```python
from build123d import *

# Parameters (mm, degrees)
ESQUISSE1_R             = 1.6
BOSS_EXTRU_1_DEPTH      = 10
ESQUISSE2_R             = 32.8
BOSS_EXTRU_2_DEPTH      = 22
ENL_V_MAT_EXTRU_1_DEPTH = 3.5
BOSS_EXTRU_3_REACH      = 79.261
ESQUISSE4_R             = 32.8
ESQUISSE5_R             = 16
BOSS_EXTRU_4_DEPTH      = 19
ESQUISSE6_R             = 1
BOSS_EXTRU_5_DEPTH      = 27
BOSS_EXTRU_6_DEPTH      = 1.5
ESQUISSE8_R             = 5
BOSS_EXTRU_7_DEPTH      = 5.5
SKETCH_1_W              = 183.813547174
SKETCH_1_H              = 124.067416174
CUT_EXTRUDE_1_DEPTH     = 18


with BuildPart() as part:
    # Esquisse1 → Boss.-Extru.1 (new body)
    with BuildSketch(Plane.XY):
        with BuildLine():
            ThreePointArc((-56.3, -16.861494596), (-60.528670487, -14.599558136), (-64.01, -11.301322931))
            ThreePointArc((-64.01, -11.301322931), (-65, 0), (-64.01, 11.301322931))
            ThreePointArc((-64.01, 11.301322931), (-60.528670487, 14.599558136), (-56.3, 16.861494596))
            Line((-56.3, 16.861494596), (-39.624688626, 23.091930519))
            ThreePointArc((-39.624688626, 23.091930519), (-36.690940127, 29.525679018), (-30.257191628, 26.591930519))
            Line((-30.257191628, 26.591930519), (-12.425, 33.254614341))
            ThreePointArc((-12.425, 33.254614341), (1.381675102, 35.473102119), (14.973963383, 32.187426436))
            Line((14.973963383, 32.187426436), (20.756023105, 34.801647207))
            ThreePointArc((20.756023105, 34.801647207), (24.347774736, 34.238511045), (26, 31))
            Line((26, 31), (25.359978077, 24.841930519))
            ThreePointArc((25.359978077, 24.841930519), (35.5, 0), (25.359978077, -24.841930519))
            Line((25.359978077, -24.841930519), (26, -31))
            ThreePointArc((26, -31), (24.347774736, -34.238511045), (20.756023105, -34.801647207))
            Line((20.756023105, -34.801647207), (14.973963383, -32.187426436))
            ThreePointArc((14.973963383, -32.187426436), (1.381675102, -35.473102119), (-12.425, -33.254614341))
            Line((-12.425, -33.254614341), (-30.257191628, -26.591930519))
            ThreePointArc((-30.257191628, -26.591930519), (-36.690940127, -29.525679018), (-39.624688626, -23.091930519))
            Line((-39.624688626, -23.091930519), (-56.3, -16.861494596))
        make_face()
        with Locations((-35, -25)):
            Circle(ESQUISSE1_R, mode=Mode.SUBTRACT)
        with Locations((22, 31)):
            Circle(ESQUISSE1_R, mode=Mode.SUBTRACT)
        with Locations((-35, 25)):
            Circle(ESQUISSE1_R, mode=Mode.SUBTRACT)
        with Locations((22, -31)):
            Circle(ESQUISSE1_R, mode=Mode.SUBTRACT)
    extrude(amount=BOSS_EXTRU_1_DEPTH)

    # Esquisse2 → Boss.-Extru.2 (add)
    with BuildSketch(Plane.XY.offset(10)):
        Circle(ESQUISSE2_R)
    extrude(amount=BOSS_EXTRU_2_DEPTH)

    # Esquisse3 → Enl_v. mat.-Extru.1 (cut)
    with BuildSketch(Plane.XY.offset(10)):
        with BuildLine():
            Line((-55.775, -15.456370046), (-37.378202776, -22.330008789))
            ThreePointArc((-37.378202776, -22.330008789), (-36.165940127, -28.120554469), (-31.453677478, -24.543603151))
            Line((-31.453677478, -24.543603151), (-11.9, -31.849489792))
            ThreePointArc((-11.9, -31.849489792), (1.664031028, -33.959255009), (14.956816294, -30.533484019))
            Line((14.956816294, -30.533484019), (21.291141631, -33.397398551))
            ThreePointArc((21.291141631, -33.397398551), (23.468656713, -33.023128137), (24.499056843, -31.06866508))
            Line((24.499056843, -31.06866508), (23.79417774, -24.286562245))
            ThreePointArc((23.79417774, -24.286562245), (34, 0), (23.79417774, 24.286562245))
            Line((23.79417774, 24.286562245), (24.499056843, 31.06866508))
            ThreePointArc((24.499056843, 31.06866508), (23.468656713, 33.023128137), (21.291141631, 33.397398551))
            Line((21.291141631, 33.397398551), (14.956816294, 30.533484019))
            ThreePointArc((14.956816294, 30.533484019), (1.664031028, 33.959255009), (-11.9, 31.849489792))
            Line((-11.9, 31.849489792), (-31.453677478, 24.543603151))
            ThreePointArc((-31.453677478, 24.543603151), (-36.165940127, 28.120554469), (-37.378202776, 22.330008789))
            Line((-37.378202776, 22.330008789), (-55.775, 15.456370046))
            ThreePointArc((-55.775, 15.456370046), (-59.496201473, 13.493411636), (-62.6, 10.653168543))
            ThreePointArc((-62.6, 10.653168543), (-63.5, 0), (-62.6, -10.653168543))
            ThreePointArc((-62.6, -10.653168543), (-59.496201473, -13.493411636), (-55.775, -15.456370046))
        make_face()
    extrude(amount=-ENL_V_MAT_EXTRU_1_DEPTH, mode=Mode.SUBTRACT)


with BuildPart() as enl_v_mat_extru_1_piece_1:
    # of the separate pieces the step leaves, piece 1, a body of its own (enl_v_mat_extru_1_pieces)
    add(part.part.solids().sort_by_distance((32.8, 0, 10))[0])


with BuildPart() as enl_v_mat_extru_1_piece_2:
    # of the separate pieces the step leaves, piece 2, a body of its own (enl_v_mat_extru_1_pieces)
    add(part.part.solids().sort_by_distance((-64.01, 11.301322931, 0))[0])

    # Esquisse4 → Boss.-Extru.3 (add, up to next)
    with BuildSketch(Plane(origin=(0, 0, 10), x_dir=(-1, 0, 0), z_dir=(0, 0, -1)), mode=Mode.PRIVATE) as boss_extru_3_sk1:
        with Locations(Location((0, 0, 0), (0, 0, 180))):
            Circle(ESQUISSE4_R)
    boss_extru_3_tool1 = extrude(boss_extru_3_sk1.sketch, amount=BOSS_EXTRU_3_REACH, mode=Mode.PRIVATE) - enl_v_mat_extru_1_piece_2.part

    add(enl_v_mat_extru_1_piece_1.part)  # Boss.-Extru.3 merges Enl_v. mat.-Extru.1 piece 1
    add(boss_extru_3_tool1.solids().sort_by_distance((0, 0, 10))[0])

    # Esquisse5 → Boss.-Extru.4 (add)
    with BuildSketch(Plane(origin=(0, 0, 0), x_dir=(-1, 0, 0), z_dir=(0, 0, -1))):
        with Locations(Location((50, 0, 0), (0, 0, 336.653490915))):
            Circle(ESQUISSE5_R)
    extrude(amount=BOSS_EXTRU_4_DEPTH)

    # Esquisse6 → Boss.-Extru.5 (add)
    # profile 1 of 4: a face of its own
    with BuildSketch(Plane(origin=(0, 0, 0), x_dir=(-1, 0, 0), z_dir=(0, 0, -1))):
        Polygon((-20.489225606, -29.008126327), (-22.969626005, -28.695694159), (-24.480400399, -30.687567832), (-23.510774394, -32.991873673), (-21.030373995, -33.304305841), (-19.519599601, -31.312432168), align=None)
        with Locations((-22, -31)):
            Circle(ESQUISSE6_R, mode=Mode.SUBTRACT)
    # profile 2 of 4: a face of its own
    with BuildSketch(Plane(origin=(0, 0, 0), x_dir=(-1, 0, 0), z_dir=(0, 0, -1))):
        Polygon((36.086835018, -22.748602735), (33.593650283, -22.933074633), (32.506815266, -25.184471898), (33.913164982, -27.251397265), (36.406349717, -27.066925367), (37.493184734, -24.815528102), align=None)
        with Locations((35, -25)):
            Circle(ESQUISSE6_R, mode=Mode.SUBTRACT)
    # profile 3 of 4: a face of its own
    with BuildSketch(Plane(origin=(0, 0, 0), x_dir=(-1, 0, 0), z_dir=(0, 0, -1))):
        Polygon((36.720274889, 26.814016072), (34.289153443, 27.396809791), (32.568878555, 25.582793719), (33.279725111, 23.185983928), (35.710846557, 22.603190209), (37.431121445, 24.417206281), align=None)
        with Locations((35, 25)):
            Circle(ESQUISSE6_R, mode=Mode.SUBTRACT)
    # profile 4 of 4: a face of its own
    with BuildSketch(Plane(origin=(0, 0, 0), x_dir=(-1, 0, 0), z_dir=(0, 0, -1))):
        Polygon((-19.952160425, 32.43399898), (-22.217959758, 33.490480585), (-24.265799333, 32.056481605), (-24.047839575, 29.56600102), (-21.782040242, 28.509519415), (-19.734200667, 29.943518395), align=None)
        with Locations((-22, 31)):
            Circle(ESQUISSE6_R, mode=Mode.SUBTRACT)
    extrude(amount=BOSS_EXTRU_5_DEPTH)

    # Esquisse7 → Boss.-Extru.6 (add)
    with BuildSketch(Plane(origin=(0, 0, -8), x_dir=(-1, 0, 0), z_dir=(0, 0, -1))):
        with BuildLine():
            Line((30.257191628, 26.591930519), (12.425, 33.254614341))
            ThreePointArc((12.425, 33.254614341), (-1.381675102, 35.473102119), (-14.973963383, 32.187426436))
            Line((-14.973963383, 32.187426436), (-20.756023105, 34.801647207))
            ThreePointArc((-20.756023105, 34.801647207), (-24.347774736, 34.238511045), (-26, 31))
            Line((-26, 31), (-25.359978077, 24.841930519))
            ThreePointArc((-25.359978077, 24.841930519), (-35.5, 0), (-25.359978077, -24.841930519))
            Line((-25.359978077, -24.841930519), (-26, -31))
            ThreePointArc((-26, -31), (-24.347774736, -34.238511045), (-20.756023105, -34.801647207))
            Line((-20.756023105, -34.801647207), (-14.973963383, -32.187426436))
            ThreePointArc((-14.973963383, -32.187426436), (-1.381675102, -35.473102119), (12.425, -33.254614341))
            Line((12.425, -33.254614341), (30.257191628, -26.591930519))
            ThreePointArc((30.257191628, -26.591930519), (36.690940127, -29.525679018), (39.624688626, -23.091930519))
            ThreePointArc((39.624688626, -23.091930519), (33.487603548, 0), (39.624688626, 23.091930519))
            ThreePointArc((39.624688626, 23.091930519), (36.690940127, 29.525679018), (30.257191628, 26.591930519))
        make_face()
    extrude(amount=BOSS_EXTRU_6_DEPTH)

    # Esquisse8 → Boss.-Extru.7 (add)
    with BuildSketch(Plane.XY.offset(6.5)):
        with Locations((-50, 0)):
            Circle(ESQUISSE8_R)
    extrude(amount=BOSS_EXTRU_7_DEPTH)

    # Sketch 1 → Cut-Extrude 1 (cut)
    with BuildSketch(Plane(origin=(0, 0, -19), x_dir=(-1, 0, 0), z_dir=(0, 0, -1))):
        with Locations((14.308056493, -2.422140446)):
            Rectangle(SKETCH_1_W, SKETCH_1_H)
    extrude(amount=CUT_EXTRUDE_1_DEPTH, mode=Mode.SUBTRACT)


solid = enl_v_mat_extru_1_piece_2.part
```
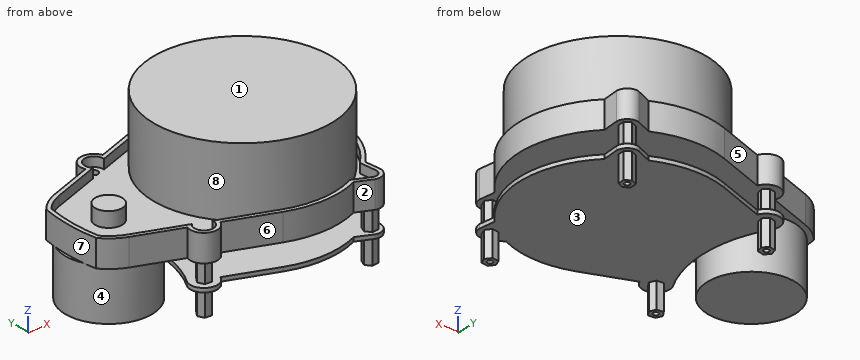
Can you work these out from the model? Positions are in its coordinate system, mm. Face numbers are marked on the shaded views. A direction names the side the tool comes from. Round coordinates to 2 decimals unless told otherwise and drop trailing zeros. Loops run counter-clockwise (first coordinate to the right, second up) from the corner with the lowest first, then second, coordinate; pieces in that order, holes last.
Item 1: Please list where these lines run through material, in increasing order: L1, parallel to Y at x = 22, z = 4; L2, parallel to Y at x = -35, z = 3.25; L3, parallel to Z at x = -27.5, y = 10.
Item 2: Suppose I cut it at A-A, the plane y = 0. Write out the boundary of the cut face in (x, z).
Item 3: Suppose I cut it at B-B, the plane x = 0.5. Write out the boundary of the cut face in (y, z), then the cut area to 3 significant figures.
Item 4: Which directions (+Z, -Z, +X, -X, +Y, -Y) give clear straight access to the entire face, cutting with the end or side of a thin tool? Please do the marked faces 4, 5, 6, 7 and 8.
Item 5: Will these pins go through, and if not, where does the flat tip stop? pin 1 Ø2 at (x, y) = (3, -18.5) entering from -Z; pin 2 Ø1 at (x, z) = (-9.5, 3.5) entering from -Y; pin 3 Ø4 at (x, y) = (-35, -25) entering from +Z.
Item 6: Suppose I cut it at C-C, the plane y = 8.5. Write out the boundary of the cut face in (x, z).
Item 7: Suppose I cut it at D-D, the plane x = -50. Write out the boundary of the cut face in (y, z).
Item 8: If we mould it in two halves opening along Y, with no side actions, what happens to the marked faces 1, 2 and 3? For each: +Y half, -Y half, draft (parallel to the pull), parting line (faces both ways), or undercut.
Reported:
1. L1: y = -35 to -32.6, -29.4 to 29.4, 32.6 to 35
1. L2: y = -29.84 to -26.6, -23.4 to 23.4, 26.6 to 29.84
1. L3: z = -9.5 to -8, 0 to 32
2. outline: (-66, -19) - (-34, -19) - (-34, 0) - (35.5, 0) - (35.5, 10) - (34, 10) - (34, 6.5) - (32.8, 6.5) - (32.8, 32) - (-32.8, 32) - (-32.8, 6.5) - (-45, 6.5) - (-45, 12) - (-55, 12) - (-55, 6.5) - (-63.5, 6.5) - (-63.5, 10) - (-65, 10) - (-65, 0) - (-66, 0) - close; (-33.49, -9.5) - (35.5, -9.5) - (35.5, -8) - (-33.49, -8) - close
3. outline: (-35.5, -9.5) - (35.5, -9.5) - (35.5, -8) - (-35.5, -8) - close; (-35.5, 0) - (35.5, 0) - (35.5, 10) - (34, 10) - (34, 6.5) - (32.8, 6.5) - (32.8, 32) - (-32.8, 32) - (-32.8, 6.5) - (-34, 6.5) - (-34, 10) - (-35.5, 10) - close
3. area: 2,250 mm2
4. face 4: -Z
4. face 5: +Z, -Z, +Y
4. face 6: +Z, -Z, -Y
4. face 7: +Z, -X
4. face 8: +Z
5. pin 1: stops at z = -9.5
5. pin 2: stops at y = -34.34
5. pin 3: stops at z = 6.5
6. outline: (-64.44, 0) - (-63.56, 0) - (-63.56, -19) - (-36.44, -19) - (-36.44, 0) - (34.47, 0) - (34.47, 10) - (32.92, 10) - (32.92, 6.5) - (31.68, 6.5) - (31.68, 32) - (-31.68, 32) - (-31.68, 6.5) - (-62.93, 6.5) - (-62.93, 10) - (-64.44, 10) - close; (-34.27, -9.5) - (34.47, -9.5) - (34.47, -8) - (-34.27, -8) - close
7. outline: (-19.22, 0) - (-16, 0) - (-16, -19) - (16, -19) - (16, 0) - (19.22, 0) - (19.22, 10) - (17.61, 10) - (17.61, 6.5) - (5, 6.5) - (5, 12) - (-5, 12) - (-5, 6.5) - (-17.61, 6.5) - (-17.61, 10) - (-19.22, 10) - close
8. face 1: draft
8. face 2: -Y half
8. face 3: undercut
